Work out the finished part from the listing and answer in its coordinate system (mm). Face numbers are marked on the shaded views. Give positions to 0.01 mm unless a question says otherwise; leave off trailing zeros. Write each loop counter-clockwise with the first axis right and the second up, starting at its lowest first coordinate (ties: lowest second). Pieces come first, ordered by that corner, then holes.
1) Find section C-C (z = 0). Determine the outline of the cut face in (x, y) (1 decimal), plus the area to 3 significant figures.
2) Determine the mould class of the marked faces 1, 2 and 3 for opening direction Z: pulls with the +Z half, pulls with the -Z half, needs draft (parallel to the pull), parting line crosses it, or undercut.
3) Find section D-D (x = -7.5). Determine the outline of the cut face in (y, z) (3 decimals).
4) Given pin 1 Ø1 at (x, z) = (-10.5, 1) entering from -Y; pin 2 Ø1.5 at (x, y) = (-9, 3) entering from +Z; pin 3 Ø0.5 at (y, z) = (4, 0) entering from -X, each flat-ended and moving along its own axis, determine where each tip first touches the part or whether it passes through.
5) Find section A-A (y = 4). Determine the outline of the cut face in (x, z) (1 decimal).
6) Straight lines are drawn through the part: probe 1 along Y at (x, z) = (-13.25, -0.4); probe 2 along Z at (x, y) = (-11, 3.7); probe 3 along X at (y, z) = (4.1, 0.05). For each, find the intervals that lie inside material, in ascending order.
Autodesk Inventor part; units mm, degrees
ref_plane "YZ Plane" through (0, 0, 0) normal (1, 0, 0) x (0, 1, 0)
ref_plane "XZ Plane" through (0, 0, 0) normal (0, 1, 0) x (-1, 0, 0)
ref_plane "XY Plane" through (0, 0, 0) normal (0, 0, 1) x (1, 0, 0)
sketch "Sketch1" plane through (0, 0, 0) normal (0, 1, 0) x (-1, 0, 0)
  arc A0 (0, -5) -> (0, 5) centre (0, 0) ccw
  line L0 (0, 5) -> (0, -5)
  dimension "d0" = 10
extrude "Extrusion1" add sketch "Sketch1" along normal blind 10
sketch "Sketch2" plane through (0, 0, 0) normal (1, 0, 0) x (0, 1, 0)
  line L0 (8.0172, -4.5) -> (8.0172, 4.5)
  line L1 (8.0172, 4.5) -> (2.5172, 4.5)
  line L2 (2.5172, -4.5) -> (0.0172, -2)
  line L3 (2.5172, 4.5) -> (0.0172, 2)
  line L4 (0.0172, -2) -> (0.0172, 2)
  line L5 (8.0172, -4.5) -> (2.5172, -4.5)
  point P0 (0, 0)
  dimension "d3" = 9
  dimension "d4" = 8
sketch "Sketch3" plane through (0, 0, 0) normal (1, 0, 0) x (0, 1, 0)
  line L0 (0, 2) -> (3, 5)
  arc A0 (3, 5) -> (0, 2) centre (1, 4) ccw
  line L1 (0, -2) -> (4, -6)
  arc A1 (0, -2) -> (4, -6) centre (1.75, -4.25) ccw
  line L2 (8.0325, 5) -> (11, 5)
  line L3 (11, 5) -> (11, -6)
  line L4 (11, -6) -> (8.0325, -6)
  line L5 (8.0325, -6) -> (8.0325, 5)
  line L6 (2.4911, 4.4911) -> (5, 7)
  line L7 (2.4911, 4.4911) -> (8.0325, 4.4911)
  arc A2 (8.0325, 4.4911) -> (5, 7) centre (7, 6.3303) ccw
  line L8 (2.4911, -4.4911) -> (8.5706, -4.4911)
  arc A3 (2.4911, -4.4911) -> (8.5706, -4.4911) centre (5.5309, -7.5041) ccw
  point P0 (0, 0)
extrude "Extrusion2" cut sketch "Sketch3" against normal through all
sketch "Sketch4" plane through (0, 0, 0) normal (0, 1, 0) x (-1, 0, 0)
  arc A0 (1.0726, -4.4911) -> (1.0726, 4.4911) centre (-1.125, 0) ccw
  arc A1 (1.0726, 4.4911) -> (1.0726, -4.4911) centre (-0.4517, 0) ccw
  point P0 (0, 0)
  point P1 (2.1976, -4.4911)
  point P2 (2.1976, 4.4911)
  dimension "d9" = 1.125
  dimension "d10" = 1.125
extrude "Extrusion3" cut sketch "Sketch4" along normal through all both and the other way through all
sketch "Sketch5" plane through (0, 0, 0) normal (1, 0, 0) x (0, 1, 0)
  line L0 (1.6, -1.2445) -> (1.6, 1.1555)
  line L1 (6.4325, 2.6911) -> (3.1125, 2.6911)
  line L2 (6.4325, -2.6911) -> (6.4325, 2.6911)
  line L3 (6.4325, -2.6911) -> (3.1125, -2.6911)
  line L4 (0, 2) -> (0, -2)
  line L5 (8.0325, 4.4911) -> (8.0325, -4.4911)
  line L6 (0, 2) -> (2.4911, 4.4911)
  line L7 (2.4911, 4.4911) -> (8.0325, 4.4911)
  line L8 (8.0325, 4.4911) -> (8.0325, -4.4911)
  line L9 (8.0325, -4.4911) -> (2.4911, -4.4911)
  line L10 (2.4911, -4.4911) -> (0, -2)
  line L11 (0, 2) -> (0, -2)
  line L12 (1.6, 1.1555) -> (3.1125, 2.6911)
  line L13 (1.6, -1.2445) -> (3.1125, -2.6911)
  line L14 (1.6, 4.6579) -> (1.6, -5.3823)
  arc A0 (1.6, 4.6579) -> (1.6, -5.3823) centre (3.2437, -0.3622) ccw
  line L15 (1.6, 1.1555) -> (5.4757, 5.0906)
  line L16 (1.6, 1.1555) -> (1.6, 7.5999)
  arc A1 (5.4757, 5.0906) -> (1.6, 7.5999) centre (3.8837, 6.8794) ccw
  line L17 (3.1125, 2.6911) -> (12.4034, 2.6911)
  line L18 (3.1125, 2.6911) -> (8.5318, 8.1936)
  arc A2 (12.4034, 2.6911) -> (8.5318, 8.1936) centre (8.3272, 3.9364) ccw
  line L19 (6.4325, 2.6911) -> (13.6333, 2.6911)
  line L20 (6.4325, 2.6911) -> (6.4325, -9.3636)
  arc A3 (6.4325, -9.3636) -> (13.6333, 2.6911) centre (6.37, -1.1482) ccw
  line L21 (6.4325, -2.6911) -> (6.4325, -11.5775)
  line L22 (6.4325, -2.6911) -> (3.1125, -2.6911)
  line L23 (3.1125, -2.6911) -> (3.2437, -12.8567)
  arc A4 (3.2437, -12.8567) -> (6.4325, -9.3636) centre (5.6123, -11.8169) ccw
  line L24 (1.6, -1.2445) -> (1.6, -8.2222)
  line L25 (1.6, -1.2445) -> (3.1125, -2.6911)
  line L26 (3.1125, -2.6911) -> (3.1946, -9.0574)
  arc A5 (1.6, -8.2222) -> (3.1946, -9.0574) centre (2.6381, -8.1801) ccw
  point P0 (0, 0)
  dimension "d16" = 1.6
  dimension "d18" = 1.6
  dimension "d21" = 1.8
  dimension "d23" = 1.8
  dimension "d24" = 2.4
  dimension "d26" = 3.32
  dimension "d27" = 3.32
extrude "Extrusion4" cut sketch "Sketch5" against normal through all contours L14 L10 L4 L6 L0 | L13 L23 L9 L10 L14 | L14 L6 L7 L15 L12 | L3 L20 L9 L23 | L14 A0 L6 L4 L10 | L10 L9 L23 A5 L24 L14 | L15 L7 L5 L17 L1 | L14 L16 A1 L15 L7 L6 | L2 L17 L5 L9 L20 | L9 L20 A4 L23 | L15 L18 A2 L17 L5 L7 | L9 L5 L17 L19 A3 L20
sketch "Sketch6" plane through (0, 0, 0) normal (1, 0, 0) x (0, 1, 0)
  circle A0 centre (4, 0) radius 1.575
  line L0 (1.6, -1.2445) -> (1.6, 1.1555)
  point P0 (0, 0)
  dimension "d31" = 3.15
  dimension "d32" = 2.4
extrude "Extrusion5" add sketch "Sketch6" against normal blind 15
sketch "Sketch7" plane through (0, 0, 0) normal (0, 1, 0) x (-1, 0, 0)
  arc A0 (3.089, -2.6911) -> (3.7176, -1.2445) centre (-1.125, 0) ccw
  arc A1 (3.7397, 1.1555) -> (3.089, 2.6911) centre (-1.125, 0) ccw
  arc A2 (3.7176, -1.2445) -> (3.7397, 1.1555) centre (-1.125, 0) ccw
  arc A3 (3.089, 2.6911) -> (3.089, -2.6911) centre (1.8078, 0) ccw
  point P0 (0, 0)
extrude "Extrusion6" cut sketch "Sketch7" along normal through all
sketch "Sketch8" plane through (-15, 4, 0) normal (-1, 0, 0) x (0, 0, 1)
  circle A0 centre (0, 0) radius 0.5375
  point P0 (0, -4)
  dimension "d37" = 1.075
extrude "Extrusion7" cut sketch "Sketch8" against normal blind 7
sketch "Sketch9" plane through (0, 0, 0) normal (0, 1, 0) x (-1, 0, 0)
  line L0 (6, 3) -> (2, 3)
  line L1 (2, 3) -> (2, -3)
  line L2 (2, -3) -> (6, -3)
  line L3 (6, -3) -> (6, 3)
  point P0 (0, 0)
extrude "Extrusion8" cut sketch "Sketch9" along normal through all both and the other way through all
properties part number "flat_cranial_window_stabilizer_Apr0119"
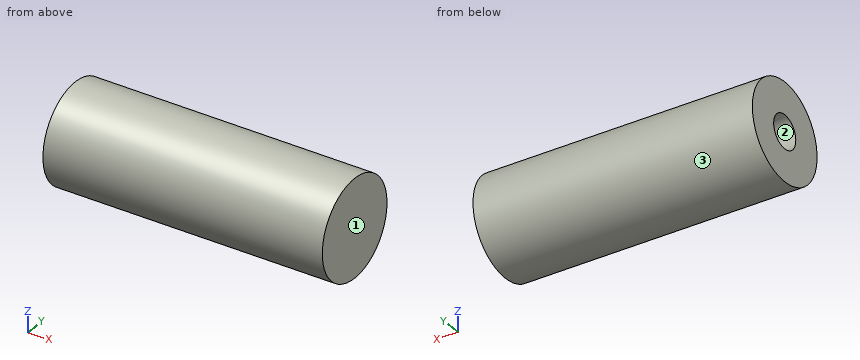
Results:
1. outline: (-15, 2.4) - (-6, 2.4) - (-6, 5.6) - (-15, 5.6) - (-15, 4.5) - (-8, 4.5) - (-8, 3.5) - (-15, 3.5) - close
1. area: 20.8 mm2
2. face 1: needs draft
2. face 2: undercut
2. face 3: parting line crosses it
3. outline: circle Ø3.15 at (4, 0)
4. pin 1: stops at y = 2.51
4. pin 2: stops at z = 1.56
4. pin 3: stops at x = -8
5. outline: (-15, -1.6) - (-6, -1.6) - (-6, 1.6) - (-15, 1.6) - (-15, 0.5) - (-8, 0.5) - (-8, -0.5) - (-15, -0.5) - close
6. probe 1: y = 2.48 to 3.64, 4.36 to 5.52
6. probe 2: z = -1.55 to -0.45, 0.45 to 1.55
6. probe 3: x = -8 to -6
